Design review of the part built by this model. Coordinates are the model's own, in mm. A direction names the side the tool comes from. Round coordinates to 2 decimals unless told otherwise and drop trailing zeros. Loops run counter-clockwise (first coordinate to the right, second up) from the corner with the lowest first, then second, coordinate; pieces in that order, holes last. Notation, with made-up numbers: (-6.75, -24) - (26.25, -24) arc R24 ccw to (26.25, 2) - close; hole circle Ø3 at (-28.75, 54). An arc over 180 degrees is marked (long way). Return JSON: item names as keys, results as strings. Group by question number.
from build123d import *

# Parameters (mm, degrees)
F0_W     = 42.3415824771
F0_H     = 39.5551770926
F0_W_2   = 39.7675335407
F0_H_2   = 41.6155532002
F1_DEPTH = 25.4
F2_W     = 35.4850441217
F2_H     = 35.8898155391
F2_W_2   = 38.453374058
F2_H_2   = 37.7787537873
F3_DEPTH = 25.4
F4_W     = 39.8773439229
F4_H     = 37.0570905507
F4_W_2   = 37.3032912612
F4_H_2   = 38.8300158083
F5_DEPTH = 25.4
F6_R     = 4.0879753591
F6_R_2   = 4.0037311952
F6_R_3   = 4.0854495617
F6_R_4   = 4.1705192674
F6_R_5   = 3.9465691335
F7_DEPTH = 25.4
F8_R     = 4.138200079
F8_R_2   = 3.8699291695
F8_R_3   = 4.1902853873
F8_R_4   = 4.3971579596
F8_R_5   = 4.0885433944
F9_DEPTH = 25.4


with BuildPart() as f1:
    # F0 (on Front) → F1 (new body)
    with BuildSketch(Plane.XZ):
        with Locations((21.1707912385, 19.7775885463)):
            Rectangle(F0_W, F0_H)
        with Locations((-19.8837667704, -20.8077766001)):
            Rectangle(F0_W_2, F0_H_2)
        with Locations((21.1707912385, -20.8077766001)):
            Rectangle(F0_W, F0_H_2)
        with Locations((-19.8837667704, 19.7775885463)):
            Rectangle(F0_W_2, F0_H)
    extrude(amount=F1_DEPTH)

    # F2 (on face) → F3 (join)
    with BuildSketch(Plane.XZ.offset(25.4)):
        with Locations((-17.7425220609, 17.9449077696)):
            Rectangle(F2_W, F2_H)
        with Locations((19.226687029, 17.9449077696)):
            Rectangle(F2_W_2, F2_H)
        with Locations((-17.7425220609, -18.8893768936)):
            Rectangle(F2_W, F2_H_2)
        with Locations((19.226687029, -18.8893768936)):
            Rectangle(F2_W_2, F2_H_2)
    extrude(amount=F3_DEPTH)

    # F4 (on face) → F5 (join)
    with BuildSketch(Plane(origin=(0, 0, 0), x_dir=(-1, 0, 0), z_dir=(0, 1, 0))):
        with Locations((-19.9386719614, 18.5285452753)):
            Rectangle(F4_W, F4_H)
        with Locations((18.6516456306, 18.5285452753)):
            Rectangle(F4_W_2, F4_H)
        with Locations((18.6516456306, -19.4150079042)):
            Rectangle(F4_W_2, F4_H_2)
        with Locations((-19.9386719614, -19.4150079042)):
            Rectangle(F4_W, F4_H_2)
    extrude(amount=F5_DEPTH)

    # F6 (on face) → F7 (join)
    with BuildSketch(Plane.YZ.offset(42.3415824771)):
        with Locations((-13.346764259, 28.1461030245)):
            Circle(F6_R)
        with Locations((-13.7779414654, 12.6237412915)):
            Circle(F6_R_2)
        with Locations((-13.346764259, -2.0362669602)):
            Circle(F6_R_3)
        with Locations((-13.346764259, -16.5525507182)):
            Circle(F6_R_4)
        with Locations((-13.6342160404, -30.9251081198)):
            Circle(F6_R_5)
    extrude(amount=F7_DEPTH)

    # F8 (on face) → F9 (join)
    with BuildSketch(Plane(origin=(-39.7675335407, 0, 0), x_dir=(0, -1, 0), z_dir=(-1, 0, 0))):
        with Locations((12.4844107777, 28.8647320122)):
            Circle(F8_R)
        with Locations((12.6281362027, 13.7735465541)):
            Circle(F8_R_2)
        with Locations((12.771862559, -1.0301880538)):
            Circle(F8_R_3)
        with Locations((12.915587984, -17.2711778432)):
            Circle(F8_R_4)
        with Locations((12.4844107777, -30.7813826948)):
            Circle(F8_R_5)
    extrude(amount=F9_DEPTH)


solid = f1.part
Q1. Add section A-A, the plane x = -29. State the section outline as (y, z) points, plus the area to 3 significant figures.
Q2. For line 1 (X direction, y = 14.5, z = -27); line 2 (Z direction, x = 12.5, y = 11); line 3 (Z direction, x = -0.5, y = -46.5), list the stretches that pass through material, from the lowest coordinate up.
Q3. Tool access review of faces 4 (the flat face through (-35.485, -38, 0)), 5 (the flat face through (1, -38, -37.779)), 6 (the cylindrical face through (54.86, -9.96, 13.83)): name each direction out of +Z, -Z, +X, -X, +Y, -Y from which nothing blocks a thin tool from reaching the whole face with its end or side.
Q4. Add section C-C, the plane y = 19. State the section outline as (x, z) points.
Q5. Insertion check: pin 1 Ø3 at (y, z) = (-5, 8.5) entering from +X; pin 2 Ø5 at (y, z) = (5.5, 0) entering from +X; pin 3 Ø20.5 at (x, y) = (2, 15.5) entering from -Z. Each pin has a flat end and moves straight along its axis. Give the tip position at first contact, or say it passes through.
Q6. Add section D-D, the plane z = -14.5. State the section outline as (x, y) points.
Q7. Draft analysis for pull direction X (two halves, no side actions). For faces 1 (the flat face through (1, 13, 37.057)), 2 (the flat face through (39.877, 13, 0)), 3 (the flat face through (-65.168, -13, 14)), state which applies: pulls with the +X half, pulls with the -X half, needs draft (parallel to the pull), parting line crosses it, or undercut.
Q8. Add section B-B, the plane x = -46. State the section outline as (y, z) points.
Evaluation:
{
 "1": {"outline": "(-50.8, -37.78) - (-25.4, -37.78) - (-25.4, -41.62) - (0, -41.62) - (0, -38.83) - (25.4, -38.83) - (25.4, 37.06) - (0, 37.06) - (0, 39.56) - (-25.4, 39.56) - (-25.4, 35.89) - (-50.8, 35.89) - close", "area": "5,860 mm²"},
 "2": {"line 1": "-37.3 to 39.88", "line 2": "-38.83 to 37.06", "line 3": "-37.78 to 35.89"},
 "3": {"face 4": "+Z, -Z, -X, -Y", "face 5": "-Z, +X, -X, -Y", "face 6": "+X"},
 "4": {"outline": "(-37.3, -38.83) - (39.88, -38.83) - (39.88, 37.06) - (-37.3, 37.06) - close"},
 "5": {"pin 1": "x = 42.34", "pin 2": "x = 39.88", "pin 3": "z = -38.83"},
 "6": {"outline": "(-65.17, -16.33) - (-39.77, -16.33) - (-39.77, -25.4) - (-35.49, -25.4) - (-35.49, -50.8) - (38.45, -50.8) - (38.45, -25.4) - (42.34, -25.4) - (42.34, -16.98) - (67.74, -16.98) - (67.74, -9.72) - (42.34, -9.72) - (42.34, 0) - (39.88, 0) - (39.88, 25.4) - (-37.3, 25.4) - (-37.3, 0) - (-39.77, 0) - (-39.77, -9.5) - (-65.17, -9.5) - close"},
 "7": {"face 1": "needs draft", "face 2": "pulls with the +X half", "face 3": "pulls with the -X half"},
 "8": {"outline": "circle Ø8.79 at (-12.92, -17.27); circle Ø8.38 at (-12.77, -1.03); circle Ø8.28 at (-12.48, 28.86); circle Ø8.18 at (-12.48, -30.78); circle Ø7.74 at (-12.63, 13.77)"}
}
